Check sheet for the drawn part. Datum: minimum x, y, z corner. Units: mm. Coordinates: 2 decimals unless noted, no trailing zeros. Order: outer loops, then holes, each group sorted by start corner. A loop starts at its lowest first (then second) coordinate and runs counter-clockwise, first axis right, second up.
Q1. Cross-section at C-C, the plane y = 13.25. Record the boundary of the cut face in (x, z).
Q2. Cross-section at B-B, the plane z = 10. Record the boundary of the cut face in (x, y), and give its area (3 significant figures).
Q3. Cross-section at A-A, the plane x = 6.5. Record the boundary of the cut face in (y, z), and give its area (3 significant figures).
Q4. Cross-section at D-D, the plane y = 2.5. Record the boundary of the cut face in (x, z).
Q5. Depth check by flat-ended pin: P1, Ø2.5, axis at x = 28.5, z = 10, coming from the -Y side. Enter the tip coordinate at first touch or a pass-through.
Q6. Thickness scan on line 1 (Z direction, x = 6.5, y = 11.5); line 2 (X direction, y = 6.5, z = 8); line 3 (X direction, y = 3, z = 9.75). Record the ranges inside material, lowest first.
Q7. Draft check along Z on the marked faces 1, 2 and 3. Enter one of: pulls with the +Z half, pulls with the -Z half, needs draft (parallel to the pull), parting line crosses it, or undercut.
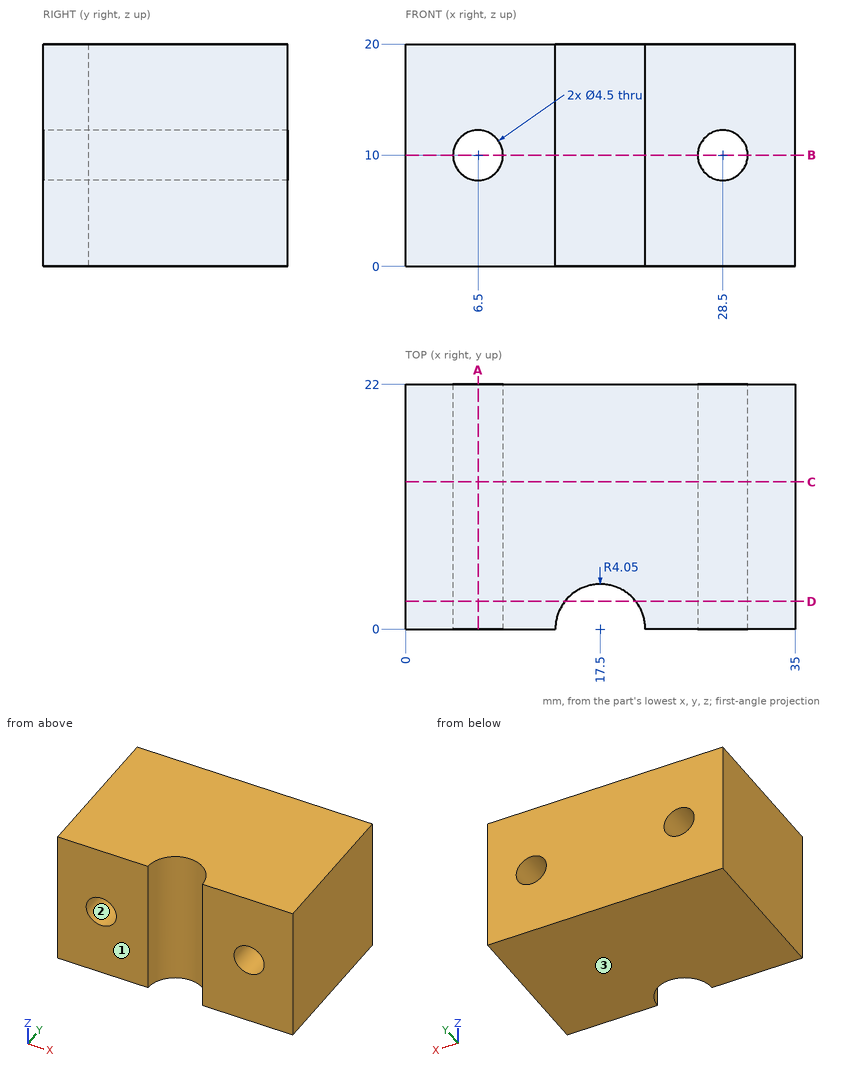
Check values:
1. outline: (0, 0) - (35, 0) - (35, 20) - (0, 20) - close; hole circle Ø4.5 at (6.5, 10); hole circle Ø4.5 at (28.5, 10)
2. outline: (0, 0) - (4.25, 0) - (4.25, 22) - (0, 22) - close; (8.75, 0) - (13.45, 0) arc R4.05 cw to (21.55, 0) - (26.25, 0) - (26.25, 22) - (8.75, 22) - close; (30.75, 0) - (35, 0) - (35, 22) - (30.75, 22) - close
2. area: 546 mm2
3. outline: (0, 0) - (22, 0) - (22, 7.75) - (0, 7.75) - close; (0, 12.25) - (22, 12.25) - (22, 20) - (0, 20) - close
3. area: 341 mm2
4. outline: (0, 0) - (14.31, 0) - (14.31, 20) - (0, 20) - close; (20.69, 0) - (35, 0) - (35, 20) - (20.69, 20) - close; hole circle Ø4.5 at (6.5, 10); hole circle Ø4.5 at (28.5, 10)
5. P1: passes through
6. line 1: z = 0 to 7.75, 12.25 to 20
6. line 2: x = 0 to 5.47, 7.53 to 27.47, 29.53 to 35
6. line 3: x = 0 to 4.26, 8.74 to 14.78, 20.22 to 26.26, 30.74 to 35
7. face 1: needs draft
7. face 2: undercut
7. face 3: pulls with the -Z half
